from build123d import *

# Parameters (mm, degrees)
SKETCH3_R            = 145
SKETCH3_R_2          = 105
SKETCH5_W            = 360
SKETCH5_H            = 360
BOSS_EXTRUDE1_DEPTH  = 50
SKETCH6_R            = 105
CUT_EXTRUDE1_DEPTH   = 50
FILLET1_R            = 20
SKETCH7_R            = 15
CUT_EXTRUDE4_DEPTH   = 50
SKETCH9_R            = 30
CUT_EXTRUDE5_DEPTH   = 10
FILLET1_OF_MIRROR3_R = 20


with BuildPart() as part:
    # Sweep1: sweep along a path in Sketch1
    with BuildLine(Plane.XY) as sweep1_path:
        Line((0, 0), (-150, 0))
        ThreePointArc((-150, 0), (-333.847763109, 76.152236891), (-410, 260))
        Line((-410, 260), (-410, 410))
    # Sketch3 → Sweep1 (sweep)
    with BuildSketch(Plane(origin=(0, 410, 0), x_dir=(1, 0, 0), z_dir=(0, 1, 0))):
        with Locations((-410, 0)):
            Circle(SKETCH3_R)
        with Locations((-410, 0)):
            Circle(SKETCH3_R_2, mode=Mode.SUBTRACT)
    sweep(path=sweep1_path.line)

    # Sketch5 → Boss-Extrude1 (add)
    with BuildSketch(Plane(origin=(0, 410, 0), x_dir=(1, 0, 0), z_dir=(0, 1, 0))):
        with Locations((-410, 0)):
            Rectangle(SKETCH5_W, SKETCH5_H)
    boss_extrude1 = extrude(amount=-BOSS_EXTRUDE1_DEPTH)

    # Sketch6 → Cut-Extrude1 (cut)
    with BuildSketch(Plane(origin=(0, 410, 0), x_dir=(1, 0, 0), z_dir=(0, 1, 0))):
        with Locations(Location((-410, 0, 0), (0, 0, 270))):
            Circle(SKETCH6_R)
    cut_extrude1 = extrude(amount=-CUT_EXTRUDE1_DEPTH, mode=Mode.SUBTRACT)

    # Fillet1
    fillet1_edges = [part.edges().sort_by_distance(p)[0] for p in [
        (-590, 385, 180),
        (-590, 385, -180),
        (-230, 385, -180),
        (-230, 385, 180),
    ]]
    fillet(fillet1_edges, radius=FILLET1_R)

    # Sketch7 → Cut-Extrude4 (cut)
    with BuildSketch(Plane(origin=(0, 410, 0), x_dir=(1, 0, 0), z_dir=(0, 1, 0))):
        with Locations(Location((-540, 130, 0), (0, 0, 270))):
            Circle(SKETCH7_R)
        with Locations(Location((-280, 130, 0), (0, 0, 90))):
            Circle(SKETCH7_R)
        with Locations(Location((-280, -130, 0), (0, 0, 270))):
            Circle(SKETCH7_R)
        with Locations(Location((-540, -130, 0), (0, 0, 90))):
            Circle(SKETCH7_R)
    cut_extrude4 = extrude(amount=-CUT_EXTRUDE4_DEPTH, mode=Mode.SUBTRACT)

    # Sketch9 → Cut-Extrude5 (cut)
    with BuildSketch(Plane(origin=(0, 410, 0), x_dir=(1, 0, 0), z_dir=(0, 1, 0))):
        with Locations(Location((-540, -130, 0), (0, 0, 270))):
            Circle(SKETCH9_R)
        with Locations(Location((-280, -130, 0), (0, 0, 270))):
            Circle(SKETCH9_R)
        with Locations(Location((-540, 130, 0), (0, 0, 270))):
            Circle(SKETCH9_R)
        with Locations(Location((-280, 130, 0), (0, 0, 270))):
            Circle(SKETCH9_R)
    cut_extrude5 = extrude(amount=-CUT_EXTRUDE5_DEPTH, mode=Mode.SUBTRACT)

    # Mirror3: Boss-Extrude1, Cut-Extrude1, Cut-Extrude4, Cut-Extrude5 across plane
    add(boss_extrude1.mirror(Plane(origin=(-205, 205, 0), x_dir=(0, 0, 1), z_dir=(-0.7071067811865475, 0.7071067811865477, 0))))
    add(cut_extrude1.mirror(Plane(origin=(-205, 205, 0), x_dir=(0, 0, 1), z_dir=(-0.7071067811865475, 0.7071067811865477, 0))), mode=Mode.SUBTRACT)
    add(cut_extrude4.mirror(Plane(origin=(-205, 205, 0), x_dir=(0, 0, 1), z_dir=(-0.7071067811865475, 0.7071067811865477, 0))), mode=Mode.SUBTRACT)
    add(cut_extrude5.mirror(Plane(origin=(-205, 205, 0), x_dir=(0, 0, 1), z_dir=(-0.7071067811865475, 0.7071067811865477, 0))), mode=Mode.SUBTRACT)

    # Fillet1 of Mirror3
    fillet1_of_mirror3_edges = [part.edges().sort_by_distance(p)[0] for p in [
        (-25, -180, 180),
        (-25, -180, -180),
        (-25, 180, -180),
        (-25, 180, 180),
    ]]
    fillet(fillet1_of_mirror3_edges, radius=FILLET1_OF_MIRROR3_R)


solid = part.part
Design review of the part built by this model. Coordinates are the model's own, in mm. A direction names the side the tool comes from. Round coordinates to 2 decimals unless told otherwise and drop trailing zeros. Loops run counter-clockwise (first coordinate to the right, second up) from the corner with the lowest first, then second, coordinate; pieces in that order, holes last. Notation, with made-up numbers: M 57,89 L 110,89 A30 ccw 110,119 Z; hole C -28.75,-27 d10. An arc over 180 degrees is marked long. Answer as a JSON object with one key per item and string values.
Item 1: Clearance check with flat-ended pins moving along their axes: P1, Ø5, axis at y = 337, z = 75.5, coming from the +X side; P2, Ø6, axis at x = -369, z = 60, coming from the +Y side; P3, Ø24, axis at x = -280, z = 130, coming from the -Y side; P4, Ø3, axis at y = -93, z = -136.5, coming from the +X side. State where each tip first meets the part, or that it passes through.
Answer sheet:
{"P1": "stops at x = -284.72", "P2": "stops at y = -4.36", "P3": "stops at y = -59.41", "P4": "stops at x = 0"}
Item 2: The part is to be moulded in two halves that separate along Z. For faces 6 (the flat face through (-546, 400, -144)), 7 (the cylindrical face through (-278.68, 405.07, -159.97)), 8 (the flat face through (0, -83, -83)), 9 (the flat face through (-412, 385, -180)), say which applies: pulls with the +Z half, pulls with the -Z half, needs draft (parallel to the pull), parting line crosses it, or undercut.
Answer sheet:
{"face 6": "undercut", "face 7": "undercut", "face 8": "needs draft", "face 9": "pulls with the -Z half"}
Item 3: We need section A-A on z = 0. Give the boundary of the cut face in (x, y).
Answer sheet:
{"outline": "M -590,360 L -555,360 L -555,260 A405 ccw -150,-145 L -50,-145 L -50,-180 L 0,-180 L 0,-105 L -150,-105 A365 cw -515,260 L -515,410 L -590,410 Z; M -305,260 A155 ccw -150,105 L 0,105 L 0,180 L -50,180 L -50,145 L -150,145 A115 cw -265,260 L -265,360 L -230,360 L -230,410 L -305,410 Z"}
Item 4: Wall thickness on L1, parallel to Z at x = -123.5, y = 0; L2, parallel to X at y = 404, z = -130; L3, parallel to Z at x = -414.5, y = 315: over which ranges is each line inside the solid? List them lowest first. Write a range as from..to.
Answer sheet:
{"L1": "z = -145..-105, 105..145", "L2": "x = -590..-570, -510..-310, -250..-230", "L3": "z = -144.93..-104.9, 104.9..144.93"}
Item 5: We need section B-B on x = -71. Give the boundary of the cut face in (y, z).
Answer sheet:
{"outline": "C 0,0 d290; hole C 0,0 d210"}
Item 6: Machinability: for faces 1 (the flat face through (-546, 400, 116)), 2 (the flat face through (-533, 360, -83)), 3 (the flat face through (-10, 124, -144)), 4 (the flat face through (-25, -2, -180)), 5 (the cylindrical face through (-25.35, -174.297, 173.986)), which of the approach directions +Z, -Z, +X, -X, +Y, -Y give a long, thin tool a straight path to every point of the face, cutting with its end or side? Answer none if there is none.
Answer sheet:
{"face 1": "+Y", "face 2": "none", "face 3": "+X", "face 4": "-Z, +X, -X, +Y, -Y", "face 5": "+Z, +X, -X, -Y"}
Item 7: We need section D-D on y = 130. State how many separate pieces and enclosed holes the cut face has, and give its area (3 significant figures).
Answer sheet:
{"separate pieces": "3", "enclosed holes": "1", "area": "71,600 mm^2"}
Item 8: We need section C-C on y = 313.5. Give the boundary of the cut face in (x, z).
Answer sheet:
{"outline": "C -410,0 d290; hole C -410,0 d210"}
